Input: part model. Units: mm. Frame: model coordinates. Coordinates: 2 decimals unless noted, no trailing zeros. Loops run counter-clockwise (first coordinate to the right, second up) from the corner with the lowest first, then second, coordinate; pieces in that order, holes last.
Item 1: Section C-C on x = 572. Return loops of the section in (y, z), and give its area (3 significant figures).
Item 2: Section D-D on y = 3.5. Return loops of the section in (x, z), and give its area (3 significant figures).
Item 3: Section A-A on x = 546. Return loops of the section in (y, z), and give its area (3 significant figures).
Item 4: Ray query, line 1 along Y through (x, z) = (543, 0.15); line 2 along Y through (x, z) = (569, 0.3); line 3 along Y through (x, z) = (587.5, 1.35). Return the intervals inside material, ascending.
Item 5: Contact query for flat-ended pins moving along their axis: P1, Ø0.9, axis at x = 565, z = 2, coming from the +Y side; P2, Ø1.5, axis at y = -31, z = 2, coming from the -X side; P3, Ø1.5, axis at x = 544, z = 1, coming from the +Y side. Output: stop coordinate, or through.
Item 6: Section B-B on z = 1.65. Return loops of the section in (x, y), and give its area (3 significant figures).
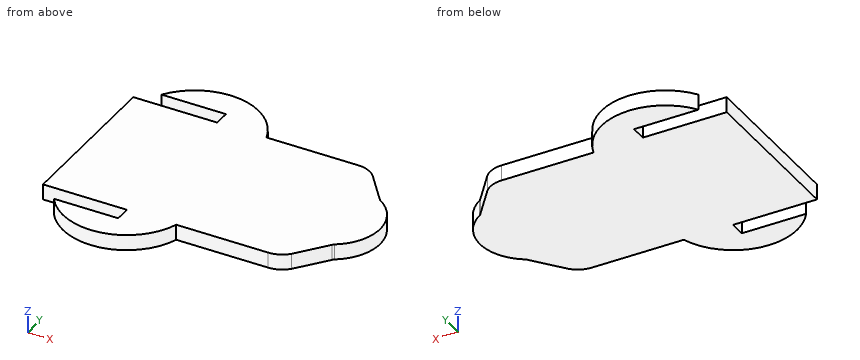
```python
from build123d import *

# Parameters (mm, degrees)
BASE_EXTRUDE_DEPTH = 3


with BuildPart() as part:
    # Sketch1 → Base-Extrude (new body)
    with BuildSketch(Plane.XY):
        with BuildLine():
            Line((534.507066227, 1.566585982), (534.507066227, -29.433414018))
            Line((534.507066227, -29.433414018), (550.643129996, -29.433414018))
            Line((550.643129996, -29.433414018), (550.643129996, -32.433414018))
            Line((550.643129996, -32.433414018), (538.258588448, -32.433414018))
            ThreePointArc((538.258588448, -32.433414018), (550.12702098, -37.759556083), (560.122161718, -29.433414018))
            Line((560.122161718, -29.433414018), (577.454155209, -29.433414018))
            Line((577.454155209, -29.433414018), (577.793445205, -29.433414018))
            ThreePointArc((577.793445205, -29.433414018), (579.752044999, -29.024576285), (581.383534897, -27.866343942))
            Line((581.383534897, -27.866343942), (585.943497105, -22.135687625))
            ThreePointArc((585.943497105, -22.135687625), (586.10909179, -21.942450413), (586.288300693, -21.761767294))
            ThreePointArc((586.288300693, -21.761767294), (590.621491518, -13.933414018), (586.288300693, -6.105060742))
            ThreePointArc((586.288300693, -6.105060742), (586.10909179, -5.924377623), (585.943497105, -5.731140411))
            Line((585.943497105, -5.731140411), (581.383534897, -0.000484094))
            ThreePointArc((581.383534897, -0.000484094), (579.752044999, 1.157748249), (577.793445205, 1.566585982))
            Line((577.793445205, 1.566585982), (577.454155209, 1.566585982))
            Line((577.454155209, 1.566585982), (560.122161718, 1.566585982))
            ThreePointArc((560.122161718, 1.566585982), (550.12702098, 9.892728047), (538.258588448, 4.566585982))
            Line((538.258588448, 4.566585982), (550.643129996, 4.566585982))
            Line((550.643129996, 4.566585982), (550.643129996, 1.566585982))
            Line((550.643129996, 1.566585982), (534.507066227, 1.566585982))
        make_face()
    extrude(amount=BASE_EXTRUDE_DEPTH)


solid = part.part
```
Results found:
1. outline: (-29.43, 0) - (1.57, 0) - (1.57, 3) - (-29.43, 3) - close
1. area: 93.0 mm2
2. outline: (550.64, 0) - (559.3, 0) - (559.3, 3) - (550.64, 3) - close
2. area: 26.0 mm2
3. outline: (-37.63, 0) - (-32.43, 0) - (-32.43, 3) - (-37.63, 3) - close; (-29.43, 0) - (1.57, 0) - (1.57, 3) - (-29.43, 3) - close; (4.57, 0) - (9.76, 0) - (9.76, 3) - (4.57, 3) - close
3. area: 124 mm2
4. line 1: y = -36.59 to -32.43, -29.43 to 1.57, 4.57 to 8.73
4. line 2: y = -29.43 to 1.57
4. line 3: y = -20.86 to -7.01
5. P1: stops at y = 1.57
5. P2: stops at x = 550.64
5. P3: stops at y = 9.43
6. outline: (534.51, -29.43) - (550.64, -29.43) - (550.64, -32.43) - (538.26, -32.43) arc R12.28 ccw to (560.12, -29.43) - (577.79, -29.43) arc R4.9 ccw to (581.38, -27.87) - (585.94, -22.14) arc R3.5 cw to (586.29, -21.76) arc R9.24 ccw to (586.29, -6.11) arc R3.5 cw to (585.94, -5.73) - (581.38, 0) arc R4.9 ccw to (577.79, 1.57) - (560.12, 1.57) arc R12.28 ccw to (538.26, 4.57) - (550.64, 4.57) - (550.64, 1.57) - (534.51, 1.57) - close
6. area: 1,810 mm2
